```python
from build123d import *

# Parameters (mm, degrees)
F0_W     = 101.6
F0_H     = 127
F1_DEPTH = 101.6
F2_W     = 50.8
F2_H     = 5.08
F3_DEPTH = 25.4
F4_W     = 12.7
F4_H     = 29.5519137372
F4_H_2   = 38.5342074425
F5_DEPTH = 5.08
F6_W     = 12.7
F6_H     = 63.5
F7_DEPTH = 5.08
F8_R     = 3.3143898489
F9_DEPTH = 109.22


with BuildPart() as f1:
    # F0 (on Front) → F1 (new body)
    with BuildSketch(Plane.XZ):
        with Locations((-50.8, 63.5)):
            Rectangle(F0_W, F0_H)
    extrude(amount=F1_DEPTH)

    # F2 (on face) → F3 (join)
    with BuildSketch(Plane.YZ):
        with Locations((-44.8094035365, 15.8326673792)):
            Rectangle(F2_W, F2_H)
    extrude(amount=F3_DEPTH)

    # F4 (on face) → F5 (join)
    with BuildSketch(Plane.XZ.offset(101.6)):
        with Locations((-57.4776338577, 141.7759568686)):
            Rectangle(F4_W, F4_H)
        with Locations((-57.4776338577, 107.7328962787)):
            Rectangle(F4_W, F4_H_2)
    extrude(amount=F5_DEPTH)

    # F6 (on face) → F7 (join)
    with BuildSketch(Plane(origin=(0, 0, 0), x_dir=(-1, 0, 0), z_dir=(0, 1, 0))):
        with Locations((57.4776338577, 124.8019137372)):
            Rectangle(F6_W, F6_H)
    extrude(amount=F7_DEPTH)

    # F8 (on face) → F9 (join)
    with BuildSketch(Plane(origin=(0, 5.08, 0), x_dir=(-1, 0, 0), z_dir=(0, 1, 0))):
        with Locations((56.3409850001, 145.4961895943)):
            Circle(F8_R)
    extrude(amount=-F9_DEPTH)


solid = f1.part
```
The listing builds one solid part. Answer for the finished solid, in the listing's coordinates (mm). A direction names the side the tool comes from. Give positions to 0.01 mm unless a question says otherwise; leave off trailing zeros. Loops run counter-clockwise (first coordinate to the right, second up) from the corner with the lowest first, then second, coordinate; pieces in that order, holes last. Notation, with made-up numbers: M 50,30.25 L 74,30.25 A14 ccw 74,46.25 Z; hole C -11,-25.75 d4. An arc over 180 degrees is marked long. One line per item, written item: value.
1. Section B-B on y = -57 is taken. Determine the outline of the cut face in (x, z), plus the area to 3 significant figures.
Found:
outline: M -101.6,0 L 0,0 L 0,13.29 L 25.4,13.29 L 25.4,18.37 L 0,18.37 L 0,127 L -101.6,127 Z; C -56.34,145.5 d6.63
area: 13,100 mm^2
2. Section D-D on x = -81.5 is taken. Determine the outline of the cut face in (y, z), plus the area to 3 significant figures.
Found:
outline: M -101.6,0 L 0,0 L 0,127 L -101.6,127 Z
area: 12,900 mm^2
3. Find the intervals of material crossed by probe 1 along Z at (x, y) = (-56, -3); probe 2 along Z at (x, y) = (-62.5, -27); probe 3 along Y at (x, z) = (-73, 54), in increasing order.
Found:
probe 1: 0 to 127, 142.2 to 148.79
probe 2: 0 to 127
probe 3: -101.6 to 0
4. For a pull along Y with two mould halves and no side action, classify faces 5 (the face through (13, -45, 18.373)), 6 (the face through (13, -70.209, 16)), 7 (the face through (-58, -101.6, 142)) as pulls with the +Y half, pulls with the -Y half, needs draft (parallel to the pull), parting line crosses it, or undercut.
Found:
face 5: needs draft
face 6: pulls with the -Y half
face 7: undercut
5. Section C-C on z = 109.5 is taken. Determine the outline of the cut face in (x, y), plus the area to 3 significant figures.
Found:
outline: M -101.6,-101.6 L -63.83,-101.6 L -63.83,-106.68 L -51.13,-106.68 L -51.13,-101.6 L 0,-101.6 L 0,0 L -51.13,0 L -51.13,5.08 L -63.83,5.08 L -63.83,0 L -101.6,0 Z
area: 10,500 mm^2
6. Section A-A on z = 133.5 is taken. Determine the outline of the cut face in (x, y), plus the area to 3 significant figures.
Found:
outline: M -63.83,-106.68 L -51.13,-106.68 L -51.13,-101.6 L -63.83,-101.6 Z; M -63.83,0 L -51.13,0 L -51.13,5.08 L -63.83,5.08 Z
area: 129 mm^2
7. Each of these flat-tipped pins is pushed along its axis until it touches: P1, Ø4, axis at x = -55.5, y = 2.5, coming from the -Z side; P2, Ø20.5, axis at x = 9.5, y = -51.5, coming from the -Z side; P3, Ø10, axis at x = -79, y = -74.5, coming from the +Z side; P4, Ø1.5, axis at x = -78.5, z = 34, coming from the +Y side. Where does it stop, or does it pass through?
Found:
P1: z = 93.05
P2: z = 0
P3: z = 127
P4: y = 0
8. For faces 1 (the face through (13, -19.409, 16)), 2 (the face through (-58, -104, 88.466)), 3 (the face through (-51.128, -104, 122)), 4 (the face through (-57.87, -50.089, 142.556)), determine the directions among +Z, -Z, +X, -X, +Y, -Y from which every point of the face is accessible in a straight line to the end or side of a thin tool.
Found:
face 1: +Z, -Z, +X, +Y
face 2: -Z, +X, -X, -Y
face 3: +Z, -Z, +X, -Y
face 4: none
